Can you work these out from the model? Positions are in its coordinate system, mm. Give positions to 0.01 mm unless a question says otherwise; leave off trailing zeros. Loops run counter-clockwise (first coordinate to the right, second up) from the corner with the lowest first, then second, coordinate; pieces in that order, holes last. Notation, with made-up numbers: (-2, 53.5) -> (9, 53.5) arc R25 cw to (9, 85.5) -> close; hole circle Ø3 at (40, -32). An arc over 180 degrees is marked (long way). Return JSON: item names as keys, results as strings. Group by question number.
Q1. I need wall thicknesses on line 1 along X through (y, z) = (30.5, 8.25); line 2 along X through (y, z) = (53.5, 9); line 3 along Y through (x, z) = (-95, 3). Which ranges of each line are inside material? Lowest first, please. Write a range as [from, to].
Q2. Suppose I cut it at D-D, the plane x = -112.5. Please give me the cut outline in (y, z), and give its area (3 significant figures).
Q3. Suppose I cut it at C-C, the plane x = -76. Please give me the cut outline in (y, z), and give its area (3 significant figures).
Q4. Suppose I cut it at B-B, the plane y = -20. Please give me the cut outline in (x, z).
Q5. Suppose I cut it at A-A, the plane x = -160. Please give me the cut outline in (y, z).
Q6. Will these pins go through, and if not, where does the flat tip stop? pin 1 (2.5 mm diameter, centred on x = 7.24, y = 45.37, fed in from -Z); pin 2 (3.5 mm diameter, centred on x = 7.06, y = -49.4, fed in from -Z); pin 3 (6 mm diameter, centred on x = -36, y = -44, fed in from +Z); pin 4 (6 mm diameter, centred on x = -193.5, z = 6, fed in from -Y).
```python
from build123d import *

# Parameters (mm, degrees)
BOSS_EXTRUDE1_DEPTH      = 10
BOSS_EXTRUDE1_DEPTH_BACK = 0.01
SKETCH7_W                = 169
SKETCH7_H                = 58
CUT_EXTRUDE4_DEPTH       = 261.116514656
SKETCH18_W               = 47.4
SKETCH18_H               = 47.4
CUT_EXTRUDE18_DEPTH      = 261.116514656
SKETCH28_W               = 4.75290021
SKETCH28_H               = 9.947843747
BOSS_EXTRUDE6_DEPTH      = 115.870057685
SKETCH30_W               = 14.12
SKETCH30_H               = 25
CUT_EXTRUDE25_DEPTH      = 4.5
SKETCH33_R               = 1.55
CUT_EXTRUDE26_DEPTH      = 10.01
SKETCH44_W               = 18
SKETCH44_H               = 2.51
CUT_EXTRUDE30_DEPTH      = 10.01


with BuildPart() as part:
    # Sketch1 → Boss-Extrude1 (new, two sides: drawn at the far end of the back side and taken through both)
    with BuildSketch(Plane.XY.offset(-BOSS_EXTRUDE1_DEPTH_BACK)):
        with BuildLine():
            Line((0, 0), (0, -37))
            Line((0, -37), (60, -37))
            Line((60, -37), (60, -52))
            Line((60, -52), (33.129942315, -78.870057685))
            Line((33.129942315, -78.870057685), (-55.850057685, -78.870057685))
            ThreePointArc((-55.850057685, -78.870057685), (-169.614041234, -90.257166815), (-239.999947532, -0.158696229))
            ThreePointArc((-239.999947532, -0.158696229), (-169.748285548, 90.207490359), (-55.850057685, 78.870057685))
            Line((-55.850057685, 78.870057685), (33.129942315, 78.870057685))
            Line((33.129942315, 78.870057685), (60, 52))
            Line((60, 52), (60, 37))
            Line((60, 37), (0, 37))
            Line((0, 37), (0, 0))
        make_face()
    extrude(amount=BOSS_EXTRUDE1_DEPTH + BOSS_EXTRUDE1_DEPTH_BACK)

    # Sketch7 → Cut-Extrude4 (cut, through all)
    with BuildSketch(Plane.XY.offset(10)):
        with Locations((-128.91309413, -19.94383898)):
            Rectangle(SKETCH7_W, SKETCH7_H)
    extrude(amount=-CUT_EXTRUDE4_DEPTH, mode=Mode.SUBTRACT)

    # Sketch18 → Cut-Extrude18 (cut, through all)
    with BuildSketch(Plane.XY.offset(10)):
        with Locations((-80.42454895, 45.3)):
            Rectangle(SKETCH18_W, SKETCH18_H)
    extrude(amount=-CUT_EXTRUDE18_DEPTH, mode=Mode.SUBTRACT)

    # Sketch28 → Boss-Extrude6 (add)
    with BuildSketch(Plane.XZ.offset(78.870057685)):
        with Locations((16.603067585, 5.033719824)):
            Rectangle(SKETCH28_W, SKETCH28_H)
    extrude(amount=-BOSS_EXTRUDE6_DEPTH)

    # Sketch30 → Cut-Extrude25 (cut)
    with BuildSketch(Plane(origin=(0, 0, -0.01), x_dir=(-1, 0, 0), z_dir=(0, 0, -1))):
        with Locations((-7.06, -49.5)):
            Rectangle(SKETCH30_W, SKETCH30_H)
        Polygon((-14.38072485, 61.935396467), (-14.275539526, 36.935617747), (-0.155664505, 36.995026418), (-0.260849829, 61.994805138), align=None)
    extrude(amount=-CUT_EXTRUDE25_DEPTH, mode=Mode.SUBTRACT)

    # Sketch33 → Cut-Extrude26 (cut)
    with BuildSketch(Plane(origin=(0, 0, -0.01), x_dir=(-1, 0, 0), z_dir=(0, 0, -1))):
        with Locations((-7.06, -53.4)):
            Circle(SKETCH33_R)
        with Locations((-7.06, -49.4)):
            Circle(SKETCH33_R)
        with Locations((-7.06, -45.4)):
            Circle(SKETCH33_R)
        with Locations((-7.06, -41.4)):
            Circle(SKETCH33_R)
        with Locations((-7.228632788, 41.370889137)):
            Circle(SKETCH33_R)
        with Locations((-7.244931474, 45.370855931)):
            Circle(SKETCH33_R)
        with Locations((-7.261230159, 49.370822725)):
            Circle(SKETCH33_R)
        with Locations((-7.277528845, 53.370789519)):
            Circle(SKETCH33_R)
    extrude(amount=-CUT_EXTRUDE26_DEPTH, mode=Mode.SUBTRACT)

    # Sketch44 → Cut-Extrude30 (cut)
    with BuildSketch(Plane(origin=(0, 0, -0.01), x_dir=(-1, 0, 0), z_dir=(0, 0, -1))):
        with Locations((20.303305502, -13.815974066)):
            Rectangle(SKETCH44_W, SKETCH44_H)
        Polygon((29.23066644, 16.565007379), (29.218146833, 19.074976156), (11.218370746, 18.985194117), (11.230890353, 16.47522534), align=None)
    extrude(amount=-CUT_EXTRUDE30_DEPTH, mode=Mode.SUBTRACT)


solid = part.part
```
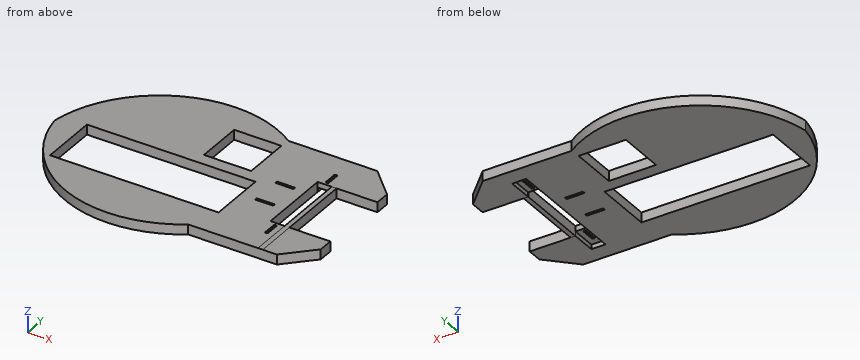
Ans:
{
 "1": {"line 1": "x = [-230.79, -104.12], [-56.72, 0], [14.23, 18.98]", "line 2": "x = [-216.97, -104.12], [-56.72, 5.73], [8.82, 58.5]", "line 3": "y = [-96.42, -48.94], [9.06, 21.6], [69, 96.43]"},
 "2": {"outline": "(-99.32, -0.01) -> (-48.94, -0.01) -> (-48.94, 10) -> (-99.32, 10) -> close; (9.06, -0.01) -> (99.33, -0.01) -> (99.33, 10) -> (9.06, 10) -> close", "area": "1,410 mm^2"},
 "3": {"outline": "(-90.04, -0.01) -> (-48.94, -0.01) -> (-48.94, 10) -> (-90.04, 10) -> close; (9.06, -0.01) -> (21.6, -0.01) -> (21.6, 10) -> (9.06, 10) -> close; (69, -0.01) -> (90.04, -0.01) -> (90.04, 10) -> (69, 10) -> close", "area": "748 mm^2"},
 "4": {"outline": "(-235.02, -0.01) -> (-213.41, -0.01) -> (-213.41, 10) -> (-235.02, 10) -> close; (-44.41, -0.01) -> (0, -0.01) -> (0, 10) -> (-44.41, 10) -> close; (14.23, 0.06) -> (18.98, 0.06) -> (18.98, 10.01) -> (14.23, 10.01) -> close"},
 "5": {"outline": "(-93.88, -0.01) -> (-48.94, -0.01) -> (-48.94, 10) -> (-93.88, 10) -> close; (9.06, -0.01) -> (93.89, -0.01) -> (93.89, 10) -> (9.06, 10) -> close"},
 "6": {"pin 1": "passes through", "pin 2": "stops at z = 4.49", "pin 3": "stops at z = 10", "pin 4": "stops at y = -78.72"}
}
